Geometry check sheet. Reference: the model listing, model coordinates, mm. A direction names the side the tool comes from. Give positions to 0.01 mm unless a question says otherwise; leave off trailing zeros. Write each loop counter-clockwise with the first axis right and the second up, starting at its lowest first coordinate (ties: lowest second). Pieces come first, ordered by that corner, then holes.
(1) Cross-section at B-B (y = 54.8). Record the boundary of the cut face in (x, z), and give its area (3 significant figures).
(2) Cross-section at C-C (x = -13.5). Record the boundary of the cut face in (y, z), and give its area (3 significant figures).
(3) Tool access check on faces 4 (the cylindrical face through (21.583, 53.33, 1.972)), 5 (the flat face through (-8.837, 28, -2)), 6 (the cylindrical face through (-19.82, 27.81, -2.22)). Record the directions out of +Z, -Z, +X, -X, +Y, -Y that give a thin tool (end or side, any length) a straight path to the whole face; none if there is none.
(4) Depth check by flat-ended pin: P1, Ø3, axis at y = 25.5, z = 2.5, coming from the +X side; P2, Ø2, axis at x = -1.2, y = 54.8, coming from the -Z side; P3, Ø1.3, axis at y = 28.5, z = -1.5, coming from the +X side; P4, Ø1.2, axis at y = 29.5, z = 2, coming from the -X side. Enter the tip coordinate at first touch or a pass-through.
(5) Cross-section at D-D (y = 16). Record the boundary of the cut face in (x, z).
(6) Mould release check, pull along X, two halves, no side actions. Record for faces 1 (the flat face through (-19.5, 28, 2)), 2 (the flat face through (32.1, 28, -2)), 3 (the flat face through (-17, 25, -4.5)): +X half, -X half, draft (parallel to the pull), parting line (faces both ways), or undercut.
(7) Cross-section at A-A (z = -3.5). Record the boundary of the cut face in (x, y), and give its area (3 significant figures).
(8) Thickness scan on line 1 along Y through (x, z) = (25.1, 3.1); line 2 along Y through (x, z) = (-1.2, 1); line 3 along X through (y, z) = (16, 3.25). Record the ranges inside material, lowest first.
```python
from build123d import *

# Parameters (mm, degrees)
CROQUIS1_W               = 22
CROQUIS1_H               = 55.2
SALIENTE_EXTRUIR1_DEPTH  = 4
CROQUIS2_W               = 12.1
CROQUIS2_H               = 4
CORTAR_EXTRUIR1_DEPTH    = 9.6
CROQUIS3_W               = 12.1
CROQUIS3_H               = 4
CORTAR_EXTRUIR2_DEPTH    = 9.6
CORTAR_EXTRUIR3_DEPTH    = 16
CORTAR_EXTRUIR4_START    = -16
CORTAR_EXTRUIR4_DEPTH    = 16
CROQUIS9_W               = 11.778481694
CROQUIS9_H               = 4
CORTAR_EXTRUIR5_DEPTH    = 2
CROQUIS11_W              = 4.95
CROQUIS11_H              = 4
SALIENTE_EXTRUIR3_DEPTH  = 2
CROQUIS12_W              = 4
CROQUIS12_H              = 1.8
SALIENTE_EXTRUIR4_DEPTH  = 12.1
CROQUIS13_W              = 4.95
CROQUIS13_H              = 4
SALIENTE_EXTRUIR5_DEPTH  = 2
CROQUIS14_W              = 4
CROQUIS14_H              = 1.8
SALIENTE_EXTRUIR6_DEPTH  = 12.1
CROQUIS17_W              = 4
CROQUIS17_H              = 59.2
SALIENTE_EXTRUIR8_DEPTH  = 11.5
CROQUIS18_W              = 4
CROQUIS18_H              = 59.2
SALIENTE_EXTRUIR9_DEPTH  = 11.5
CROQUIS19_R              = 1.75
CORTAR_EXTRUIR6_DEPTH    = 11.5
CROQUIS27_W              = 12.1
CROQUIS27_H              = 55.6
CORTAR_EXTRUIR8_DEPTH    = 10
CROQUIS28_W              = 12.1
CROQUIS28_H              = 4
SALIENTE_EXTRUIR10_DEPTH = 55.6
CROQUIS33_W              = 4
CROQUIS33_H              = 59.2
SALIENTE_EXTRUIR13_DEPTH = 8
CROQUIS30_R              = 2.1
CORTAR_EXTRUIR9_DEPTH    = 10
CROQUIS32_W              = 4
CROQUIS32_H              = 59.2
SALIENTE_EXTRUIR12_DEPTH = 8
SALIENTE_EXTRUIR11_DEPTH = 4.5
CORTAR_EXTRUIR10_DEPTH   = 8


with BuildPart() as part:
    # Croquis1 → Saliente-Extruir1 (new body)
    with BuildSketch(Plane.XY):
        with Locations((11, 27.6)):
            Rectangle(CROQUIS1_W, CROQUIS1_H)
    extrude(amount=SALIENTE_EXTRUIR1_DEPTH)

    # Croquis2 → Cortar-Extruir1 (cut)
    with BuildSketch(Plane(origin=(0, 55.2, 0), x_dir=(1, 0, 0), z_dir=(0, 1, 0))):
        with Locations((11, -2)):
            Rectangle(CROQUIS2_W, CROQUIS2_H)
    extrude(amount=-CORTAR_EXTRUIR1_DEPTH, mode=Mode.SUBTRACT)

    # Croquis3 → Cortar-Extruir2 (cut)
    with BuildSketch(Plane.XZ):
        with Locations((11, 2)):
            Rectangle(CROQUIS3_W, CROQUIS3_H)
    extrude(amount=-CORTAR_EXTRUIR2_DEPTH, mode=Mode.SUBTRACT)

    # Croquis5 → Cortar-Extruir3 (cut)
    with BuildSketch(Plane.XZ.offset(-9.6)):
        with BuildLine():
            Line((7.4, 4), (14.6, 4))
            ThreePointArc((14.6, 4), (16.401151853, 1.506649462), (17.05, -1.5))
            Line((17.05, -1.5), (4.95, -1.5))
            ThreePointArc((4.95, -1.5), (5.598848147, 1.506649462), (7.4, 4))
        make_face()
    extrude(amount=-CORTAR_EXTRUIR3_DEPTH, mode=Mode.SUBTRACT)

    # Croquis7 → Cortar-Extruir4 (cut)
    with BuildSketch(Plane(origin=(0, 45.6, 0), x_dir=(1, 0, 0), z_dir=(0, 1, 0)).offset(CORTAR_EXTRUIR4_START)):
        with BuildLine():
            Line((4.95, 1.5), (17.05, 1.5))
            ThreePointArc((17.05, 1.5), (16.401151853, -1.506649462), (14.6, -4))
            Line((14.6, -4), (7.4, -4))
            ThreePointArc((7.4, -4), (5.598848147, -1.506649462), (4.95, 1.5))
        make_face()
    extrude(amount=CORTAR_EXTRUIR4_DEPTH, mode=Mode.SUBTRACT)

    # Croquis9 → Cortar-Extruir5 (cut)
    with BuildSketch(Plane(origin=(0, 0, 0), x_dir=(-1, 0, 0), z_dir=(0, 0, -1))):
        with Locations((-11, 27.6)):
            Rectangle(CROQUIS9_W, CROQUIS9_H)
    extrude(amount=-CORTAR_EXTRUIR5_DEPTH, mode=Mode.SUBTRACT)

    # Croquis11 → Saliente-Extruir3 (add)
    with BuildSketch(Plane(origin=(0, 55.2, 0), x_dir=(1, 0, 0), z_dir=(0, 1, 0))):
        with Locations((2.475, -2)):
            Rectangle(CROQUIS11_W, CROQUIS11_H)
        with Locations((19.525, -2)):
            Rectangle(CROQUIS11_W, CROQUIS11_H)
    extrude(amount=SALIENTE_EXTRUIR3_DEPTH)

    # Croquis12 → Saliente-Extruir4 (add)
    with BuildSketch(Plane(origin=(4.95, 0, 0), x_dir=(0, 0, -1), z_dir=(1, 0, 0))):
        with Locations((-2, 56.3)):
            Rectangle(CROQUIS12_W, CROQUIS12_H)
    extrude(amount=SALIENTE_EXTRUIR4_DEPTH)

    # Croquis13 → Saliente-Extruir5 (add)
    with BuildSketch(Plane.XZ):
        with Locations((19.525, 2)):
            Rectangle(CROQUIS13_W, CROQUIS13_H)
        with Locations((2.475, 2)):
            Rectangle(CROQUIS13_W, CROQUIS13_H)
    extrude(amount=SALIENTE_EXTRUIR5_DEPTH)

    # Croquis14 → Saliente-Extruir6 (add)
    with BuildSketch(Plane(origin=(4.95, 0, 0), x_dir=(0, 0, -1), z_dir=(1, 0, 0))):
        with Locations((-2, -1.1)):
            Rectangle(CROQUIS14_W, CROQUIS14_H)
    extrude(amount=SALIENTE_EXTRUIR6_DEPTH)

    # Croquis17 → Saliente-Extruir8 (add)
    with BuildSketch(Plane.ZY):
        with Locations((2, 27.6)):
            Rectangle(CROQUIS17_W, CROQUIS17_H)
    extrude(amount=SALIENTE_EXTRUIR8_DEPTH)

    # Croquis18 → Saliente-Extruir9 (add)
    with BuildSketch(Plane(origin=(22, 0, 0), x_dir=(0, 0, -1), z_dir=(1, 0, 0))):
        with Locations((-2, 27.6)):
            Rectangle(CROQUIS18_W, CROQUIS18_H)
    extrude(amount=SALIENTE_EXTRUIR9_DEPTH)

    # Croquis19 → Cortar-Extruir6 (cut)
    with BuildSketch(Plane(origin=(0, 0, 0), x_dir=(-1, 0, 0), z_dir=(0, 0, -1))):
        with Locations((-23.2, 54)):
            Circle(CROQUIS19_R)
        with Locations((1.2, 54.8)):
            Circle(CROQUIS19_R)
        with Locations((1.2, 0.5)):
            Circle(CROQUIS19_R)
        with Locations((-23.2, 0.5)):
            Circle(CROQUIS19_R)
    extrude(amount=-CORTAR_EXTRUIR6_DEPTH, mode=Mode.SUBTRACT)

    # Croquis27 → Cortar-Extruir8 (cut)
    with BuildSketch(Plane(origin=(0, 0, 0), x_dir=(-1, 0, 0), z_dir=(0, 0, -1))):
        with Locations((-11, 27.6)):
            Rectangle(CROQUIS27_W, CROQUIS27_H)
    extrude(amount=-CORTAR_EXTRUIR8_DEPTH, mode=Mode.SUBTRACT)

    # Croquis28 → Saliente-Extruir10 (add)
    with BuildSketch(Plane.XZ.offset(-55.4)):
        with Locations((11, 2)):
            Rectangle(CROQUIS28_W, CROQUIS28_H)
    extrude(amount=SALIENTE_EXTRUIR10_DEPTH)

    # Croquis33 → Saliente-Extruir13 (add)
    with BuildSketch(Plane.ZY.offset(11.5)):
        with Locations((2, 27.6)):
            Rectangle(CROQUIS33_W, CROQUIS33_H)
    extrude(amount=SALIENTE_EXTRUIR13_DEPTH)

    # Croquis30 → Cortar-Extruir9 (cut)
    with BuildSketch(Plane(origin=(0, 0, 0), x_dir=(-1, 0, 0), z_dir=(0, 0, -1))):
        with Locations((-25.1, 37.194789274)):
            Circle(CROQUIS30_R)
        with Locations((-25.1, 16.925277734)):
            Circle(CROQUIS30_R)
        with Locations((3.1, 37.194789274)):
            Circle(CROQUIS30_R)
        with Locations((3.1, 16.925277734)):
            Circle(CROQUIS30_R)
    extrude(amount=-CORTAR_EXTRUIR9_DEPTH, mode=Mode.SUBTRACT)

    # Croquis32 → Saliente-Extruir12 (add)
    with BuildSketch(Plane(origin=(33.5, 0, 0), x_dir=(0, 0, -1), z_dir=(1, 0, 0))):
        with Locations((-2, 27.6)):
            Rectangle(CROQUIS32_W, CROQUIS32_H)
    extrude(amount=SALIENTE_EXTRUIR12_DEPTH)

    # Croquis29 → Saliente-Extruir11 (add)
    with BuildSketch(Plane(origin=(0, 0, 0), x_dir=(-1, 0, 0), z_dir=(0, 0, -1))):
        with BuildLine():
            Line((-32.099895832, 32.201901781), (-32.099895832, 22.998098219))
            Line((-32.099895832, 22.998098219), (-32.099895832, 22.27255299))
            ThreePointArc((-32.099895832, 22.27255299), (-41.82, 27.6), (-32.099895832, 32.92744701))
            Line((-32.099895832, 32.92744701), (-32.099895832, 32.201901781))
        make_face()
        with BuildLine():
            Line((8.83711623, 23.32791238), (8.83711623, 31.87208762))
            ThreePointArc((8.83711623, 31.87208762), (19.824019109, 27.6), (8.83711623, 23.32791238))
        make_face()
    extrude(amount=SALIENTE_EXTRUIR11_DEPTH)

    # Croquis35 → Cortar-Revolución1 (revolve, cut)
    with BuildSketch(Plane(origin=(0, 0, -7.5), x_dir=(-1, 0, 0), z_dir=(0, 0, -1))):
        with BuildLine():
            Line((-35.5, 32.6), (-35.5, 22.6))
            ThreePointArc((-35.5, 22.6), (-40.5, 27.6), (-35.5, 32.6))
        make_face()
    revolve(axis=Axis((35.5, 32.6, -7.5), (0, -1, 0)), mode=Mode.SUBTRACT)

    # Croquis36 → Cortar-Revolución2 (revolve, cut)
    with BuildSketch(Plane(origin=(0, 0, -7.5), x_dir=(-1, 0, 0), z_dir=(0, 0, -1))):
        with BuildLine():
            Line((13.5, 32.6), (13.5, 22.6))
            ThreePointArc((13.5, 22.6), (18.5, 27.6), (13.5, 32.6))
        make_face()
    revolve(axis=Axis((-13.5, 32.6, -7.5), (0, -1, 0)), mode=Mode.SUBTRACT)

    # Croquis37 → Cortar-Extruir10 (cut)
    with BuildSketch(Plane.XY.offset(4)):
        Polygon((-19.5, 57.2), (-19.5, 34.2), (-4.5, 57.2), align=None)
        Polygon((41.5, 57.2), (26.5, 57.2), (41.5, 34.2), align=None)
        Polygon((-19.5, -2), (-19.5, 21), (-4.5, -2), align=None)
        Polygon((41.5, -2), (41.5, 21), (26.5, -2), align=None)
    extrude(amount=-CORTAR_EXTRUIR10_DEPTH, mode=Mode.SUBTRACT)


solid = part.part
```
Reply:
1. outline: (-6.07, 0) - (-2.95, 0) - (-2.95, 4) - (-6.07, 4) - close; (0.55, 0) - (21.64, 0) - (21.64, 4) - (0.55, 4) - close; (24.76, 0) - (28.07, 0) - (28.07, 4) - (24.76, 4) - close
1. area: 110 mm2
2. outline: (11.8, 0) - (21.28, 0) - (21.28, -4.5) - (23.6, -4.5) arc R5 cw to (31.6, -4.5) - (33.92, -4.5) - (33.92, 0) - (43.4, 0) - (43.4, 4) - (11.8, 4) - close
2. area: 172 mm2
3. face 4: +Z, -Z
3. face 5: -Z, +Y, -Y
3. face 6: -Z
4. P1: stops at x = 41.5
4. P2: passes through
4. P3: stops at x = 41.82
4. P4: stops at x = -19.5
5. outline: (-16.24, 0) - (-4.99, 0) - (-4.99, 4) - (-16.24, 4) - close; (-1.21, 0) - (23.21, 0) - (23.21, 4) - (-1.21, 4) - close; (26.99, 0) - (38.24, 0) - (38.24, 4) - (26.99, 4) - close
6. face 1: -X half
6. face 2: undercut
6. face 3: draft
7. outline: (-8.84, 23.33) - (-8.84, 31.87) arc R6.32 ccw (long way) to start; (32.1, 22.27) arc R6.32 ccw (long way) to (32.1, 32.93) - close; hole circle Ø6 at (-13.5, 27.6); hole circle Ø6 at (35.5, 27.6)
7. area: 163 mm2
8. line 1: y = -2 to 14.83, 19.03 to 35.09, 39.29 to 57.2
8. line 2: y = -2 to -1.25, 2.25 to 16.03, 17.82 to 36.3, 38.09 to 53.05, 56.55 to 57.2
8. line 3: x = -16.24 to -4.99, -1.21 to 23.21, 26.99 to 38.24
